Job drawing, mm, ordinate dimensions from the low corner. One solid piece. A direction names the side the tool comes from. Give positions to 0.01 mm unless a question says otherwise; leave off trailing zeros. Loops run counter-clockwise (first coordinate to the right, second up) from the corner with the lowest first, then second, coordinate; pieces in that order, holes last. Notation, with made-up numbers: M 82,3.5 L 130,3.5 A24 ccw 130,31.5 Z; hole C 36,-14 d11. An arc over 180 degrees is marked long. Answer as CSV lines item,"result".
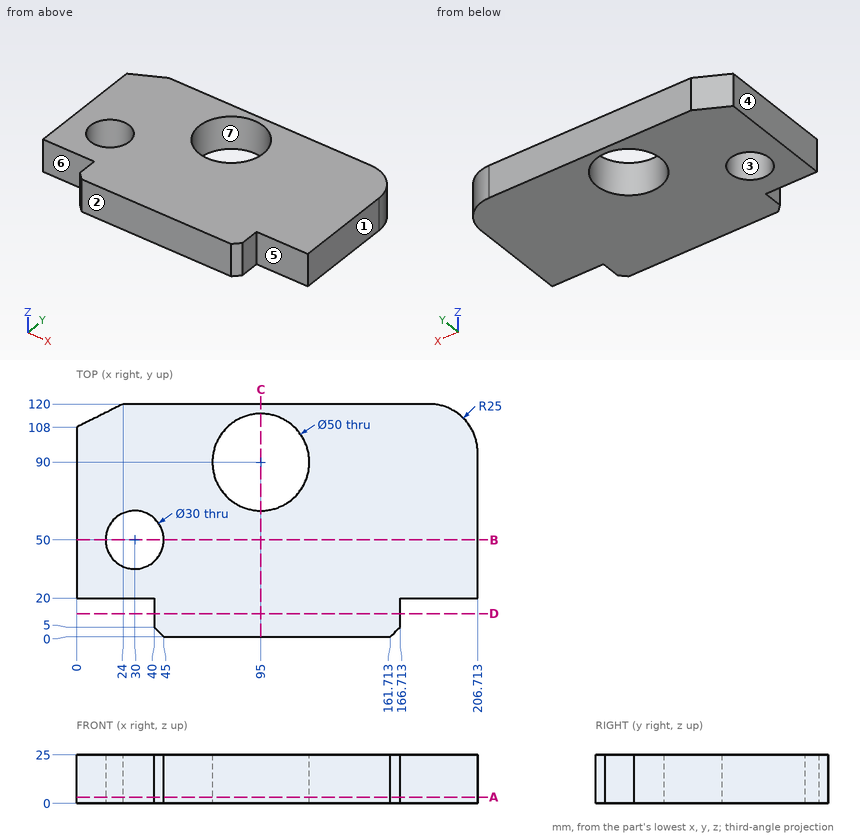
1) Flat gauge pins, fed straight in: pin 1 (12 mm diameter, centred on y = 10.5, z = 10, fed in from -X); pin 2 (12 mm diameter, centred on y = 12.5, z = 17.5, fed in from +X); pin 3 (7.5 mm diameter, centred on x = 190, z = 17, fed in from -Y); pin 4 (5 mm diameter, centred on x = 77, y = 101.5, fed in from -Z). Where does each tip first touch, or does it go through?
Answer below:
pin 1,"stops at x = 40"
pin 2,"stops at x = 166.71"
pin 3,"stops at y = 20"
pin 4,"passes through"
2) Which spindle directions (+Z, -Z, +X, -X, +Y, -Y) get a long thin tool onto all of the face, cutting with end or side? Do the marked faces 5, 6 and 7. Say none if no direction does.
Answer below:
face 5,"+Z, -Z, +X, -Y"
face 6,"+Z, -Z, -X, -Y"
face 7,"+Z, -Z"
3) Band-saw the part on B-B on y = 50. Give the cut face in (x, z), and give its area (3 significant figures).
Answer below:
outline,"M 0,0 L 15,0 L 15,25 L 0,25 Z; M 45,0 L 206.71,0 L 206.71,25 L 45,25 Z"
area,"4,420 mm^2"
4) Band-saw the part on A-A on z = 3.25. Give the cut face in (x, y), and give its area (3 significant figures).
Answer below:
outline,"M 0,20 L 40,20 L 40,5 L 45,0 L 161.71,0 L 166.71,5 L 166.71,20 L 206.71,20 L 206.71,95 A25 ccw 181.71,120 L 24,120 L 0,108 Z; hole C 30,50 d30; hole C 95,90 d50"
area,"20,200 mm^2"
5) Band-saw the part on C-C on x = 95. Give the cut face in (y, z), and give its area (3 significant figures).
Answer below:
outline,"M 0,0 L 65,0 L 65,25 L 0,25 Z; M 115,0 L 120,0 L 120,25 L 115,25 Z"
area,"1,750 mm^2"
6) Mould opens along X. For the marked faces 1, 2, 3 and 4 say: +X half, -X half, draft (parallel to the pull), parting line (faces both ways), or undercut.
Answer below:
face 1,"+X half"
face 2,"draft"
face 3,"undercut"
face 4,"-X half"
7) Band-saw the part on D-D on y = 12. Give the cut face in (x, z).
Answer below:
outline,"M 40,0 L 166.71,0 L 166.71,25 L 40,25 Z"
8) Drill centre lines: line 1 (Y direction, x = 95, z = 7.25); line 2 (Y direction, x = 30, z = 10.5); line 3 (X direction, y = 100, z = 8). Where is each one in solid material? Low to high. Write a range as from..to.
Answer below:
line 1,"y = 0..65, 115..120"
line 2,"y = 20..35, 65..120"
line 3,"x = 0..72.09, 117.91..206.21"
